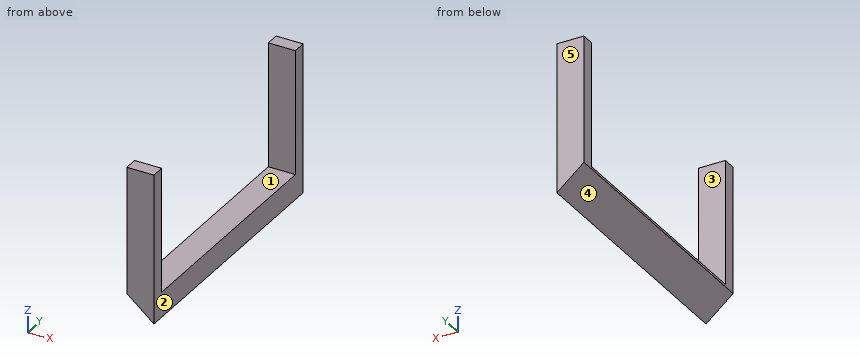
```python
from build123d import *

# Parameters (mm, degrees)
BOX016_W               = 5
BOX016_H               = 96
BOX016_DEPTH           = 60
BOX016_PLACEMENT_ANGLE = 310
BOX015_W               = 5
BOX015_H               = 96
BOX015_DEPTH           = 60
BOX015_PLACEMENT_ANGLE = 310
BOX014_W               = 5
BOX014_H               = 86
BOX014_DEPTH           = 2
BOX011_W               = 5
BOX011_H               = 86
BOX011_DEPTH           = 24
BOX006_W               = 10
BOX006_H               = 86
BOX006_DEPTH           = 20
BOX005_W               = 5
BOX005_H               = 86
BOX005_DEPTH           = 49
BOX003_W               = 10
BOX003_H               = 96
BOX003_DEPTH           = 49
BOX007_W               = 10
BOX007_H               = 96
BOX007_DEPTH           = 10


with BuildPart() as cube016:
    # Box016 → Box016 (new body)
    with BuildSketch(Plane.XY):
        with Locations((2.5, 48)):
            Rectangle(BOX016_W, BOX016_H)
    extrude(amount=BOX016_DEPTH)


with BuildPart() as cube016_1:
    # Box016 placement: moved
    add(cube016.part.moved(Location((70, 2, -56))).rotate(Axis((70, 2, -56), (0, 1, 0)), BOX016_PLACEMENT_ANGLE))


with BuildPart() as cube015:
    # Box015 → Box015 (new body)
    with BuildSketch(Plane.XY):
        with Locations((2.5, 48)):
            Rectangle(BOX015_W, BOX015_H)
    extrude(amount=BOX015_DEPTH)


with BuildPart() as cube015_1:
    # Box015 placement: moved
    add(cube015.part.moved(Location((70, 2, -59))).rotate(Axis((70, 2, -59), (0, 1, 0)), BOX015_PLACEMENT_ANGLE))


with BuildPart() as cube014:
    # Box014 → Box014 (new body)
    with BuildSketch(Plane(origin=(55, 7, -36), x_dir=(1, 0, 0), z_dir=(0, 0, 1))):
        with Locations((2.5, 43)):
            Rectangle(BOX014_W, BOX014_H)
    extrude(amount=BOX014_DEPTH)


with BuildPart() as cube011:
    # Box011 → Box011 (new body)
    with BuildSketch(Plane(origin=(40, 7, -34), x_dir=(1, 0, 0), z_dir=(0, 0, 1))):
        with Locations((2.5, 43)):
            Rectangle(BOX011_W, BOX011_H)
    extrude(amount=BOX011_DEPTH)


with BuildPart() as cube006:
    # Box006 → Box006 (new body)
    with BuildSketch(Plane(origin=(40, 7, -10), x_dir=(1, 0, 0), z_dir=(0, 0, 1))):
        with Locations((5, 43)):
            Rectangle(BOX006_W, BOX006_H)
    extrude(amount=BOX006_DEPTH)


with BuildPart() as cube005:
    # Box005 → Box005 (new body)
    with BuildSketch(Plane(origin=(45, 7, -39), x_dir=(1, 0, 0), z_dir=(0, 0, 1))):
        with Locations((2.5, 43)):
            Rectangle(BOX005_W, BOX005_H)
    extrude(amount=BOX005_DEPTH)


with BuildPart() as cut007:
    # Box003 → Box003 (new body)
    with BuildSketch(Plane(origin=(40, 2, -39), x_dir=(1, 0, 0), z_dir=(0, 0, 1))):
        with Locations((5, 48)):
            Rectangle(BOX003_W, BOX003_H)
    extrude(amount=BOX003_DEPTH)

    # Cut: cut Cube005
    add(cube005.part, mode=Mode.SUBTRACT)

    # Cut001: cut Cube006
    add(cube006.part, mode=Mode.SUBTRACT)

    # Cut004: cut Cube011
    add(cube011.part, mode=Mode.SUBTRACT)


with BuildPart() as cut007_1:
    # Cut004 placement: moved
    add(cut007.part.moved(Location((15, 0, 0))))

    # Cut007: cut Cube014
    add(cube014.part, mode=Mode.SUBTRACT)


with BuildPart() as cut009:
    # Box007 → Box007 (new body)
    with BuildSketch(Plane(origin=(55, 2, -46), x_dir=(1, 0, 0), z_dir=(0, 0, 1))):
        with Locations((5, 48)):
            Rectangle(BOX007_W, BOX007_H)
    extrude(amount=BOX007_DEPTH)

    # Fusion: union Cut007
    add(cut007_1.part)

    # Cut008: cut Cube015
    add(cube015_1.part, mode=Mode.SUBTRACT)

    # Cut009: cut Cube016
    add(cube016_1.part, mode=Mode.SUBTRACT)


solid = cut009.part
```
Input: part model. Units: mm. Frame: model coordinates. Face numbers are marked on the shaded views. A direction names the side the tool comes from. Coordinates: 2 decimals unless noted, no trailing zeros. Order: outer loops, then holes, each group sorted by start corner. A loop starts at its lowest first (then second) coordinate and runs counter-clockwise, first axis right, second up. Notation, with made-up numbers: (88, 34.25) - (95, 34.25) arc R22 cw to (95, 69.25) - close; hole circle Ø5 at (70.25, 16.25). An arc over 180 degrees is marked (long way). Return JSON: item names as keys, results as strings.
Q1. Access query for the marked faces 1 and 2. Directions: +Z, -Z, +X, -X, +Y, -Y. A direction counts if a zero-diameter tool reaches every point of the face in a straight line with its end or side. Return the directions, or none.
The answers:
{"face 1": "+Z, +X, -X", "face 2": "+Z, -Z, +X, +Y, -Y"}
Q2. Cut plane A-A (z = -33.5). Return loops of the section in (x, y), then the cut area to 3 significant figures.
The answers:
{"outline": "(55, 2) - (65, 2) - (65, 7) - (55, 7) - close; (55, 93) - (65, 93) - (65, 98) - (55, 98) - close", "area": "100 mm2"}
Q3. Cut plane D-D (x = 63). Return loops of the section in (y, z), then the cut area to 3 significant figures.
The answers:
{"outline": "(2, -43.6) - (98, -43.6) - (98, 10) - (93, 10) - (93, -36) - (7, -36) - (7, 10) - (2, 10) - close", "area": "1,190 mm2"}
Q4. Cut plane B-B (x = 56.5). Return loops of the section in (y, z), then the cut area to 3 significant figures.
The answers:
{"outline": "(2, -38.15) - (98, -38.15) - (98, 10) - (93, 10) - (93, -36) - (7, -36) - (7, 10) - (2, 10) - close", "area": "666 mm2"}
Q5. Ray query, probe 1 along Y at (x, z) = (57.75, -3); probe 2 along Z at (x, y) = (56.25, 55.5); probe 3 along Z at (x, y) = (61.75, 36.5). Return the intervals inside material, ascending.
The answers:
{"probe 1": "y = 2 to 7, 93 to 98", "probe 2": "z = -37.94 to -36", "probe 3": "z = -42.55 to -36"}
Q6. Draft query along Y for the marked faces 3, 4 and 5. Return one class per face: +Y half, -Y half, draft (parallel to the pull), parting line (faces both ways), or undercut.
The answers:
{"face 3": "undercut", "face 4": "draft", "face 5": "+Y half"}
Q7. Cut plane C-C (y = 33.5). Return loops of the section in (x, z).
The answers:
{"outline": "(55, -36.89) - (65, -45.28) - (65, -36) - (55, -36) - close"}
Q8. First-contact query: pin 1 (1.5 mm diameter, centred on x = 60, y = 81.5, fed in from -Z); pin 2 (3 mm diameter, centred on x = 61.5, y = 63.5, fed in from +Z); pin 3 (1.5 mm diameter, centred on x = 58, y = 49, fed in from -Z); pin 4 (10 mm diameter, centred on y = 84.5, z = -0.5, fed in from +X). Flat tips, straight axial feed; report the tip coordinate or a pass-through.
The answers:
{"pin 1": "stops at z = -41.71", "pin 2": "stops at z = -36", "pin 3": "stops at z = -40.03", "pin 4": "passes through"}
